The model under review builds one solid part; all positions refer to its coordinate system, in mm. Face numbers are marked on the shaded views. Round coordinates to 2 decimals unless told otherwise and drop trailing zeros. Order: outer loops, then holes, each group sorted by start corner. A loop starts at its lowest first (then second) coordinate and runs counter-clockwise, first axis right, second up. Notation, with made-up numbers: M 38,43.5 L 74,43.5 A31 ccw 74,82.5 Z; hole C -28.5,68.5 d11. An arc over 180 degrees is marked long. Answer as a JSON object with one key per item and string values. Group by question number.
1. To check wall thickness, follow probe 1 along Y at (x, z) = (102, 141); probe 2 along Z at (x, y) = (113.5, 15); probe 3 along X at (y, z) = (3.7, -101.6). State the ranges of each line that lie inside material, in increasing order. Write a range as [from, to].
2. Mouldability with a two-part tool opening along Z and no side actions: class the marked faces 1 and 2 as released by +Z, released by -Z, zero draft, split by the parting line, or undercut.
3. Add section A-A on x = -115. State the section outline as (y, z) points.
4. Add section C-C on y = 31.5. Give the number of separate pieces and of enclosed holes in the cut face, and give its area (3 significant figures).
5. Add section B-B on z = -140. State the section outline as (x, y) points, and give its area (3 significant figures).
6. Clearance check with flat-ended pins moving along their axes: P1, Ø7, axis at y = 95, z = -127.5, coming from the +X side; P2, Ø4.5, axis at x = -100, y = 79, coming from the -Z side; P3, Ø6, axis at x = -77, z = 98, coming from the +Y side. State where each tip first meets the part, or that it passes through.
7. Add section D-D on x = -82.5. State the section outline as (y, z) points, and give its area (3 significant figures).
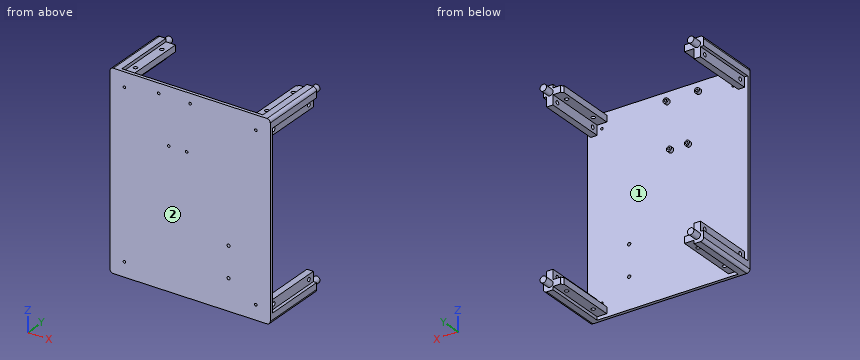
Autodesk Inventor part; units mm, degrees
ref_plane "YZ Plane" through (0, 0, 0) normal (1, 0, 0) x (0, 1, 0)
ref_plane "XZ Plane" through (0, 0, 0) normal (0, 1, 0) x (-1, 0, 0)
ref_plane "XY Plane" through (0, 0, 0) normal (0, 0, 1) x (1, 0, 0)
sketch "Sketch1" plane through (0, 0, 0) normal (0, 1, 0) x (-1, 0, 0)
  line L0 (0, 0) -> (0, 150)
  line L1 (0, 150) -> (0, -150)
  line L2 (0, -150) -> (125, -150)
  line L3 (125, -150) -> (125, 150)
  line L4 (125, 150) -> (-125, 150)
  line L5 (-125, 150) -> (-125, -150)
  line L6 (-125, -150) -> (0, -150)
  dimension "d0" = 150
  dimension "d1" = 300
  dimension "d2" = 125
  dimension "d3" = 300
  dimension "d4" = 250
  dimension "d5" = 300
extrude "Extrusion1" add sketch "Sketch1" along normal blind 5
fillet "Fillet1" radius 5 1 edges at (125, 2.5, 150)
fillet "Fillet2" radius 5 3 edges at (125, 2.5, -150) (-125, 2.5, -150) (-125, 2.5, 150)
sketch "Sketch2" plane through (0, 5, 0) normal (0, 1, 0) x (1, 0, 0)
  line L0 (120, 150) -> (-120, 150)
  line L1 (-120, 150) -> (-110, 150)
  line L2 (-110, 150) -> (-110, 145)
  line L3 (-110, 145) -> (-101.6, 145)
  arc A0 (-120, 150) -> (-125, 145) centre (-120, 145) ccw
  line L4 (-125, 145) -> (-125, 135)
  line L5 (-125, 145) -> (-125, -145)
  line L6 (-125, 135) -> (-120, 135)
  line L7 (-120, 135) -> (-120, 120)
  line L8 (-110, 145) -> (-95, 145)
  arc A1 (-120, 150) -> (-125, 145) centre (-120, 145) ccw
  line L9 (125, -145) -> (125, 145)
  line L10 (125, 0) -> (-125, 0)
  line L11 (0, 150) -> (0, -150)
  line L12 (-120, -150) -> (120, -150)
  line L13 (-95, 145) -> (-95, 135)
  line L14 (-120, 120) -> (-110, 120)
  line L15 (-95, 135) -> (-110, 135)
  line L16 (-110, 135) -> (-110, 120)
  line L17 (-120, -150) -> (-110, -150)
  line L18 (-110, -150) -> (-110, -145)
  line L19 (-125, -145) -> (-125, -135)
  line L20 (-125, -135) -> (-120, -135)
  line L21 (-120, -135) -> (-120, -120)
  line L22 (-110, -145) -> (-95, -145)
  arc A2 (-125, -145) -> (-120, -150) centre (-120, -145) ccw
  line L23 (-95, -145) -> (-95, -135)
  line L24 (-120, -120) -> (-110, -120)
  line L25 (-95, -135) -> (-110, -135)
  line L26 (-110, -135) -> (-110, -120)
  line L27 (-120, 150) -> (120, 150)
  line L28 (110, 150) -> (110, 145)
  line L29 (125, 145) -> (125, -145)
  line L30 (125, 135) -> (120, 135)
  line L31 (120, 135) -> (120, 120)
  line L32 (110, 145) -> (95, 145)
  arc A3 (125, 145) -> (120, 150) centre (120, 145) ccw
  line L33 (120, -150) -> (-120, -150)
  line L34 (95, 145) -> (95, 135)
  line L35 (120, 120) -> (110, 120)
  line L36 (95, 135) -> (110, 135)
  line L37 (110, 135) -> (110, 120)
  line L38 (95, -135) -> (110, -135)
  line L39 (95, -145) -> (95, -135)
  line L40 (110, -150) -> (110, -145)
  line L41 (120, -150) -> (110, -150)
  arc A4 (120, -150) -> (125, -145) centre (120, -145) ccw
  line L42 (125, -135) -> (120, -135)
  line L43 (120, -135) -> (120, -120)
  line L44 (120, -120) -> (110, -120)
  line L45 (110, -135) -> (110, -120)
  line L46 (110, -145) -> (95, -145)
  point P0 (0, 0)
  point P1 (-101.6, -145)
  dimension "d10" = 10
  dimension "d11" = 5
  dimension "d12" = 10
  dimension "d13" = 5
  dimension "d14" = 15
  dimension "d15" = 15
  dimension "d17" = 10
  dimension "d18" = 10
extrude "Extrusion2" add sketch "Sketch2" along normal blind 100 contours A3 L9 L30 L31 L35 L37 L36 L34 L32 L28 L0 | L2 L3 L8 L13 L15 L16 L14 L7 L6 L4 A0 L0 | L9 A4 L12 L40 L46 L39 L38 L45 L44 L43 L42 | L20 L21 L24 L26 L25 L23 L22 L18 L12 A2 L5
sketch "Sketch3" plane through (0, 105, 0) normal (0, 1, 0) x (1, 0, 0)
  line L0 (120, 150) -> (-120, 150)
  line L1 (0, 150) -> (0, -150)
  line L2 (-120, -150) -> (120, -150)
  line L3 (0, 0) -> (125, 0)
  line L4 (125, -135) -> (125, 135)
  line L5 (0, 0) -> (-125, 0)
  line L6 (-125, 135) -> (-125, -135)
  line L7 (95, 145) -> (95, 135)
  line L8 (95, 145) -> (95, 140)
  line L9 (95, 140) -> (125, 140)
  line L10 (110, 120) -> (120, 120)
  line L11 (120, 120) -> (115, 120)
  line L12 (115, 120) -> (115, 140)
  circle A0 centre (115, 140) radius 5
  circle A1 centre (115, -140) radius 5
  circle A2 centre (-115, 140) radius 5
  circle A3 centre (-115, -140) radius 5
extrude "Extrusion3" add sketch "Sketch3" along normal blind 15
sketch "Sketch4" plane through (-120, 5, -135) normal (-1, 0, 0) x (0, 0, 1)
  line L0 (15, 100) -> (0, 100)
  line L1 (0, 100) -> (7.5, 100)
  line L2 (7.5, 100) -> (7.5, 90)
  line L3 (7.5, 90) -> (7.5, 10)
  point P0 (135, -5)
  dimension "d23" = 7.5
  dimension "d24" = 10
  dimension "d25" = 80
hole "Hole1" at (-120, 95, -127.5) at (-120, 15, -127.5) direction (1, 0, 0) diameter 6 end through all
sketch "Sketch5" plane through (-120, 5, 120) normal (-1, 0, 0) x (0, 0, 1)
  line L0 (15, 100) -> (0, 100)
  line L1 (0, 100) -> (7.5, 100)
  line L2 (7.5, 100) -> (7.5, 90)
  line L3 (7.5, 90) -> (7.5, 10)
  point P0 (-120, -5)
  dimension "d35" = 10
  dimension "d36" = 80
hole "Hole2" at (-120, 95, 127.5) at (-120, 15, 127.5) direction (1, 0, 0) diameter 6 end through all
sketch "Sketch6" plane through (-110, 5, 145) normal (0, 0, 1) x (1, 0, 0)
  line L0 (0, 0) -> (0, 100)
  line L1 (0, 100) -> (7.5, 100)
  line L2 (15, 100) -> (0, 100)
  line L3 (7.5, 100) -> (7.5, 80)
  line L4 (7.5, 80) -> (7.5, 20)
  line L5 (220, 0) -> (220, 100)
  line L6 (220, 100) -> (212.5, 100)
  line L7 (205, 100) -> (220, 100)
  line L8 (212.5, 100) -> (212.5, 80)
  line L9 (212.5, 80) -> (212.5, 20)
  point P0 (110, -5)
  dimension "d44" = 20
  dimension "d45" = 60
hole "Hole3" at (-102.5, 85, 145) at (-102.5, 25, 145) direction (0, 0, -1) diameter 6 end through all
sketch "Sketch7" plane through (95, 5, 145) normal (0, 0, 1) x (1, 0, 0)
  line L0 (0, 100) -> (7.5, 100)
  line L1 (0, 100) -> (15, 100)
  line L2 (7.5, 100) -> (7.5, 80)
  line L3 (7.5, 80) -> (7.5, 20)
  point P0 (-95, -5)
  dimension "d53" = 20
  dimension "d54" = 60
hole "Hole4" at (95, 105, 145) at (102.5, 85, 145) at (102.5, 25, 145) direction (0, 0, -1) diameter 6 end through all
sketch "Sketch8" plane through (0, 5, 0) normal (0, 1, 0) x (1, 0, 0)
  line L0 (-120, -150) -> (120, -150)
  line L1 (0, -150) -> (0, -135)
  line L2 (0, -135) -> (80.9625, -135)
  line L3 (80.9625, -135) -> (-82.55, -135)
  line L4 (0, -135) -> (-49, -135)
  line L5 (-49, -135) -> (-49, -62.9)
  line L6 (0, -135) -> (0, -62.9)
  line L7 (-49, -62.9) -> (-33.376, -62.9)
  line L8 (-33.376, -62.9) -> (-5.467, -62.9)
  line L9 (-5.467, -62.9) -> (0, -62.9)
  circle A0 centre (0, -135) radius 2
  circle A1 centre (-49, -135) radius 2
  circle A2 centre (-5.467, -62.9) radius 2
  circle A3 centre (-33.376, -62.9) radius 2
  circle A4 centre (-5.467, -62.9) radius 4
  circle A5 centre (-33.376, -62.9) radius 4
  circle A6 centre (-49, -135) radius 4
  circle A7 centre (0, -135) radius 4
  point P0 (0, 0)
  dimension "d62" = 15
  dimension "d63" = 49
  dimension "d64" = 72.1
  dimension "d67" = 15.624
  dimension "d68" = 27.909
  dimension "d69" = 4
  dimension "d70" = 4
  dimension "d71" = 4
  dimension "d72" = 4
  dimension "d73" = 8
  dimension "d74" = 8
  dimension "d75" = 8
  dimension "d76" = 8
extrude "Extrusion4" add sketch "Sketch8" along normal blind 5 contours A7 L3 A0 L1 | L1 A0 L2 A7 | A7 L6 A0 L3 | L2 A0 L6 A7 | A6 L3 A1 | L3 A1 L5 A6 | L5 A1 L3 A6 | A4 L8 A2 L9 | L9 A2 L8 A4 | A5 L8 A3 L7 | L7 A3 L8 A5
sketch "Sketch9" plane through (-5.467, 5, 62.9) normal (0, 1, 0) x (1, 0, 0)
  circle A0 centre (0, 0) radius 2
  circle A1 centre (0, 0) radius 2
  circle A2 centre (5.467, -72.1) radius 4
  circle A3 centre (5.467, -72.1) radius 2
  circle A4 centre (-43.533, -72.1) radius 2
  circle A5 centre (-43.533, -72.1) radius 2
  circle A6 centre (-27.909, 0) radius 2
  circle A7 centre (-27.909, 0) radius 2
  point P0 (5.467, 62.9)
  dimension "d79" = 4
  dimension "d80" = 4
  dimension "d81" = 4
  dimension "d82" = 4
extrude "Extrusion5" cut sketch "Sketch9" against normal blind 10 contours A0 | A3 | A4 | A6
sketch "Sketch10" plane through (0, 5, 0) normal (0, 1, 0) x (1, 0, 0)
  line L0 (0, 0) -> (0, 101.6)
  line L1 (0, 101.6) -> (60, 101.6)
  line L2 (60, 101.6) -> (60, 54.1)
  circle A0 centre (60, 101.6) radius 2.5
  circle A1 centre (60, 54.1) radius 2.5
  dimension "d85" = 60
  dimension "d86" = 47.5
  dimension "d87" = 5
  dimension "d88" = 5
extrude "Extrusion6" cut sketch "Sketch10" against normal blind 10
sketch "Sketch11" plane through (0, 5, 0) normal (0, 1, 0) x (1, 0, 0)
  line L0 (-110, 120) -> (-110, 135)
  line L1 (-110, 135) -> (-110, 127.5)
  line L2 (-110, 135) -> (-95, 135)
  line L3 (-95, 135) -> (-95, 127.5)
  line L4 (-95, 127.5) -> (-110, 127.5)
  line L5 (-95, 127.5) -> (-102.5, 127.5)
  line L6 (125, -135) -> (125, 135)
  line L7 (125, 0) -> (-125, 0)
  line L8 (-125, 135) -> (-125, -135)
  line L9 (110, 150) -> (-110, 150)
  line L10 (0, 150) -> (0, -150)
  line L11 (-120, -150) -> (120, -150)
  circle A0 centre (-102.5, 127.5) radius 2
  circle A1 centre (-102.5, -127.5) radius 2
  circle A2 centre (102.5, 127.5) radius 2
  circle A3 centre (102.5, -127.5) radius 2
  point P0 (0, 0)
  dimension "d91" = 4
extrude "Extrusion7" cut sketch "Sketch11" against normal blind 15 contours A0 L4 | L4 A0 | A1 | A2 | A3
properties part number "Bottom"
Recorded:
{
 "1": {"probe 1": "y = [0, 22.04], [27.96, 82.04], [87.96, 105]", "probe 2": "z = [-150, -130.5], [-124.5, -120], [120, 124.5], [130.5, 150]", "probe 3": "x = [-125, 57.5], [62.5, 125]"},
 "2": {"face 1": "undercut", "face 2": "zero draft"},
 "3": {"outline": "M 0,-150 L 105,-150 L 105,-145 L 120,-145 L 120,-135 L 105,-135 L 105,-120 L 5,-120 L 5,120 L 105,120 L 105,135 L 120,135 L 120,145 L 105,145 L 105,150 L 0,150 Z; hole C 15,-127.5 d6; hole C 15,127.5 d6; hole C 95,-127.5 d6; hole C 95,127.5 d6"},
 "4": {"separate pieces": "4", "enclosed holes": "0", "area": "2,080 mm²"},
 "5": {"outline": "M -125,0 L 125,0 L 125,105 L 120,105 L 120,120 L 110,120 L 110,105 L 98,105 A3 cw 95,102 L 95,5 L -95,5 L -95,105 L -110,105 L -110,120 L -120,120 L -120,105 L -125,105 Z; hole C -102.5,25 d6; hole C -102.5,85 d6; hole C 102.5,25 d6; hole C 102.5,85 d6", "area": "7,430 mm²"},
 "6": {"P1": "stops at x = 120", "P2": "stops at z = -145", "P3": "stops at y = 5"},
 "7": {"outline": "M 0,-150 L 5,-150 L 5,150 L 0,150 Z", "area": "1,500 mm²"}
}
